Design review of the part built by this model. Coordinates are the model's own, in mm. Face numbers are marked on the shaded views. Coordinates: 2 decimals unless noted, no trailing zeros. Write each loop counter-clockwise with the first axis right and the second up, starting at its lowest first coordinate (ties: lowest second). Pieces come first, ordered by that corner, then holes. Notation, with made-up numbers: M -16.5,73.5 L 24.5,73.5 A15 cw 24.5,99.5 Z; hole C 34.5,-23 d9. An arc over 180 degrees is marked long. Write item = value, one per line.
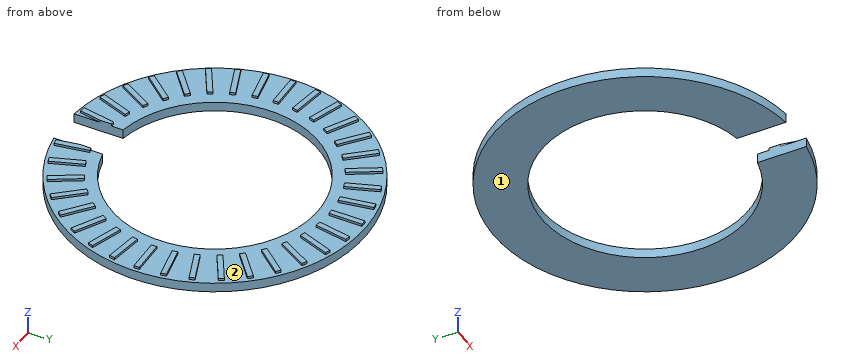
```python
from build123d import *

# Parameters (mm, degrees)
ESQUISSE1_R                  = 31.5
ESQUISSE1_R_2                = 21.5
BOSS_EXTRU_1_DEPTH           = 2
ESQUISSE2_W                  = 1.11033496
ESQUISSE2_H                  = 6.867457902
BOSS_EXTRU_2_DEPTH           = 0.5
R_P_TITION_CIRCULAIRE1_COUNT = 36
ENL_V_MAT_EXTRU_4_DEPTH      = 1.5
ENL_V_MAT_EXTRU_4_DEPTH_BACK = 3


with BuildPart() as part:
    # Esquisse1 → Boss.-Extru.1 (new body)
    with BuildSketch(Plane.XY):
        Circle(ESQUISSE1_R)
        Circle(ESQUISSE1_R_2, mode=Mode.SUBTRACT)
    extrude(amount=BOSS_EXTRU_1_DEPTH)

    # Esquisse2 → Boss.-Extru.2 (add)
    with BuildSketch(Plane.XY.offset(2)):
        with Locations((0, 27.30701826)):
            Rectangle(ESQUISSE2_W, ESQUISSE2_H)
    boss_extru_2 = extrude(amount=BOSS_EXTRU_2_DEPTH)

    # Répétition circulaire1: Boss.-Extru.2 ×36 about axis
    r_p_tition_circulaire1_axis = Axis((0, 0, 0), (0, 0, 1))
    for i in range(1, R_P_TITION_CIRCULAIRE1_COUNT):
        add(boss_extru_2.rotate(r_p_tition_circulaire1_axis, i * 360 / R_P_TITION_CIRCULAIRE1_COUNT))

    # Esquisse3 → Enlèv. mat.-Extru.4 (cut, two sides)
    with BuildSketch(Plane.XY.offset(2)) as enl_v_mat_extru_4_sk:
        Polygon((0, 0), (-4, 0), (-4, -36.523437731), (0, -36.523437731), (4, -36.523437731), (4, 0), align=None)
    extrude(amount=ENL_V_MAT_EXTRU_4_DEPTH, mode=Mode.SUBTRACT)
    extrude(enl_v_mat_extru_4_sk.sketch, amount=-ENL_V_MAT_EXTRU_4_DEPTH_BACK, mode=Mode.SUBTRACT)


solid = part.part
```
Q1. The part is to be moulded in two halves that separate along X. For the marked faces 1 and 2, say which applies: +X half, -X half, draft (parallel to the pull), parting line (faces both ways), or undercut.
Check result:
face_1 = draft
face_2 = undercut
Q2. Consider section A-A, the plane z = 1.1. State the section outline as (x, y) points (3 decimals), and give its area (3 significant figures).
Check result:
outline = M -4,-31.245 L -4,-21.125 A21.5 cw long 4,-21.125 L 4,-31.245 A31.5 ccw long Z
area = 1,580 mm²
Q3. Wall thickness on line 1 (X direction, y = 0, z = 0.7); line 2 (X direction, y = 21.5, z = 2.35); line 3 (X direction, y = -20, z = 2.15): over which ranges is each line inside the solid? List them lowest first.
Check result:
line_1 = -31.5 to -21.5, 21.5 to 31.5
line_2 = -18.77 to -17.32, -13.05 to -11.77, 11.77 to 13.05, 17.32 to 18.77
line_3 = -23.35 to -22.97, -17.51 to -16.06, 16.06 to 17.51, 22.97 to 23.35
Q4. For P1, Ø0.6, axis at x = 0, z = 2.5, coming from the -Y side; P2, Ø0.6, axis at x = 26, z = 2.5, coming from the +Y side; P3, Ø0.6, axis at y = 0, z = 2.5, coming from the +X side, all flat-tipped, find the tip position at first contact; note any pin that passes through.
Check result:
P1 = 23.87
P2 = 15.83
P3 = 30.74
